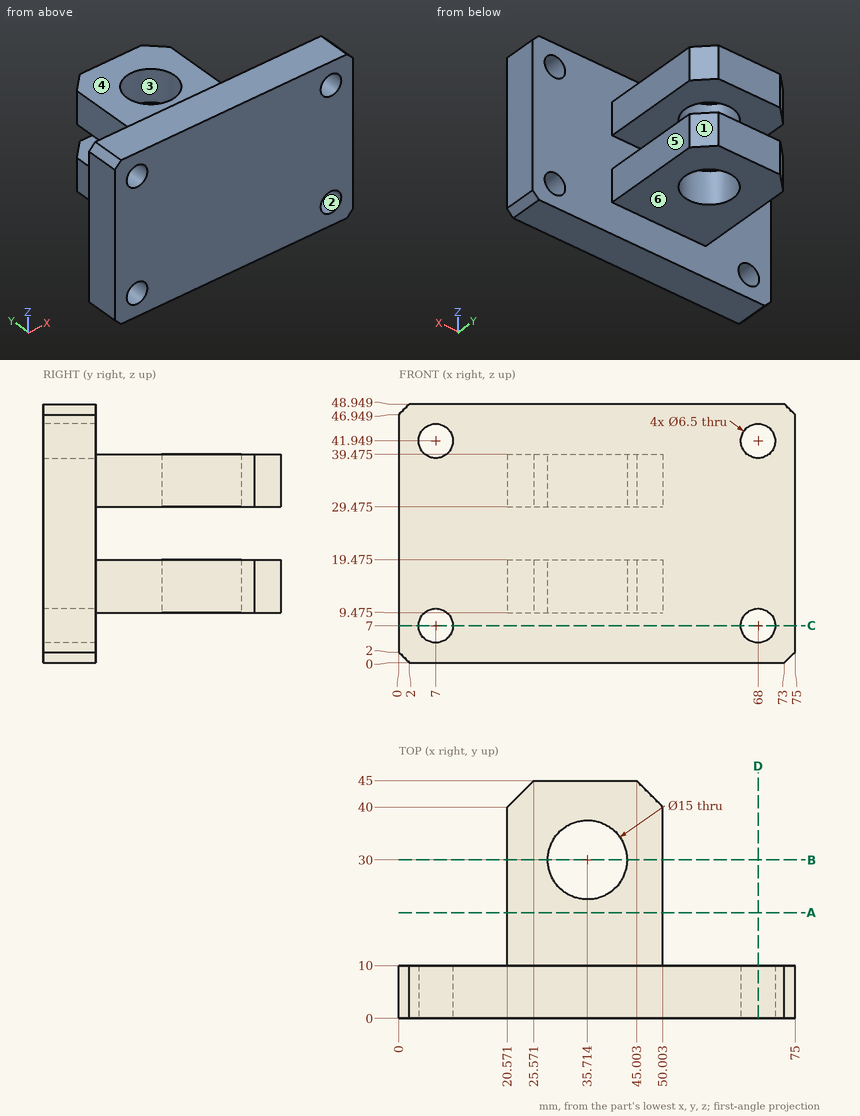
Geometry check sheet. Reference: drawing and pictorial views, mm from the part's lowest x, y, z. A direction names the side the tool comes from. Coordinates: 2 decimals unless noted, no trailing zeros. Order: outer loops, then holes, each group sorted by start corner. A loop starts at its lowest first (then second) coordinate and runs counter-clockwise, first axis right, second up.
Item 1: Mould release check, pull along Y, two halves, no side actions. Record for the marked faces 1, 2 and 3: released by +Y, released by -Y, zero draft, split by the parting line, or undercut.
Item 2: Tool access check on the marked faces 4, 5 and 6. Record the directions out of +Z, -Z, +X, -X, +Y, -Y that give a thin tool (end or side, any length) a straight path to the whole face; none if there is none.
Item 3: Section check C-C (z = 7). Enter the section's corners in (x, y).
Item 4: Scan lines: line 1 along X through (y, z) = (5, 43.5) (1 decimal); line 2 along Z through (x, y) = (21.5, 26) (1 decimal); line 3 along Y through (x, z) = (32, 4). Record each from-to range of solid material in increasing order.
Item 5: Section check A-A (y = 20). Enter the section's corners in (x, z) (1 decimal), plus the area to 3 significant figures.
Item 6: Section check B-B (y = 30). Enter the section's corners in (x, z) (1 decimal).
Item 7: Depth check by flat-ended pin: pin 1 (5 mm diameter, centred on y = 22, z = 33, fed in from -X); pin 2 (7.5 mm diameter, centred on x = 68, z = 7, fed in from +Y); pin 3 (12 mm diameter, centred on x = 28, z = 15.5, fed in from -Y); pin 4 (1.5 mm diameter, centred on y = 14, z = 38.5, fed in from +X). Enter the tip coordinate at first touch or a pass-through.
Item 8: Section check D-D (x = 68). Enter the section's corners in (y, z).
Check sheet entries:
1. face 1: released by +Y
1. face 2: zero draft
1. face 3: undercut
2. face 4: +Z, +X, -X, +Y
2. face 5: +Z, -Z, +X, +Y
2. face 6: -Z, +X, -X, +Y
3. outline: (0, 0) - (3.75, 0) - (3.75, 10) - (0, 10) - close; (10.25, 0) - (64.75, 0) - (64.75, 10) - (10.25, 10) - close; (71.25, 0) - (75, 0) - (75, 10) - (71.25, 10) - close
4. line 1: x = 0 to 4.1, 9.9 to 65.1, 70.9 to 75
4. line 2: z = 9.5 to 19.5, 29.5 to 39.5
4. line 3: y = 0 to 10
5. outline: (20.6, 9.5) - (50, 9.5) - (50, 19.5) - (20.6, 19.5) - close; (20.6, 29.5) - (50, 29.5) - (50, 39.5) - (20.6, 39.5) - close
5. area: 589 mm2
6. outline: (20.6, 9.5) - (28.2, 9.5) - (28.2, 19.5) - (20.6, 19.5) - close; (20.6, 29.5) - (28.2, 29.5) - (28.2, 39.5) - (20.6, 39.5) - close; (43.2, 9.5) - (50, 9.5) - (50, 19.5) - (43.2, 19.5) - close; (43.2, 29.5) - (50, 29.5) - (50, 39.5) - (43.2, 39.5) - close
7. pin 1: stops at x = 20.57
7. pin 2: stops at y = 10
7. pin 3: stops at y = 0
7. pin 4: stops at x = 50
8. outline: (0, 0) - (10, 0) - (10, 3.75) - (0, 3.75) - close; (0, 10.25) - (10, 10.25) - (10, 38.7) - (0, 38.7) - close; (0, 45.2) - (10, 45.2) - (10, 48.95) - (0, 48.95) - close
